Could you check a few things on this drawing? It's one solid part, dimensions in mm from its lowest x, y, z. A direction names the side the tool comes from. Give positions to 0.01 mm unless a question says otherwise; leave off trailing zeros. Write each loop counter-clockwise with the first axis right and the second up, starting at its lowest first coordinate (ties: lowest second). Pieces come first, ordered by that corner, then holes.
1. I'm going to push flat-ended pins straight in: pin 1 (5 mm diameter, centred on y = 19, z = 5, fed in from +X); pin 2 (1.5 mm diameter, centred on x = 4.5, z = 21, fed in from -Y); pin 3 (2 mm diameter, centred on x = 22.43, z = 25.97, fed in from -Y); pin 4 (0.8 mm diameter, centred on x = 5.5, y = 23.5, fed in from +Z) (1 decimal). Where does each tip first touch, or does it pass through?
2. On a 3-axis mill with a long thin cutter (end or side, diameter ignored), from which of +Z, -Z, +X, -X, +Y, -Y can I reach the whole of each face in a straight line? I mean the marked faces 1, 2 and 3. Say none if no direction works.
3. Thinking about a two-plate mould opening in X: for the marked faces 4, 5 and 6, which applies, pulls with the +X half, pulls with the -X half, needs draft (parallel to the pull), parting line crosses it, or undercut?
4. If I drill on probe 1 along Y at (x, z) = (1.5, 18.5); probe 2 along Y at (x, z) = (27.25, 16); probe 3 along Z at (x, y) = (15, 16.5), over which ranges is the centre line in solid material (lowest first)?
5. Suppose I cut it at C-C (z = 23). Please give me the cut outline in (x, y).
6. Suppose I cut it at B-B (x = 18). Please give me the cut outline in (y, z).
7. Suppose I cut it at A-A (z = 15). Please give me the cut outline in (x, y).
8. Suppose I cut it at D-D (y = 13). Please give me the cut outline in (x, z).
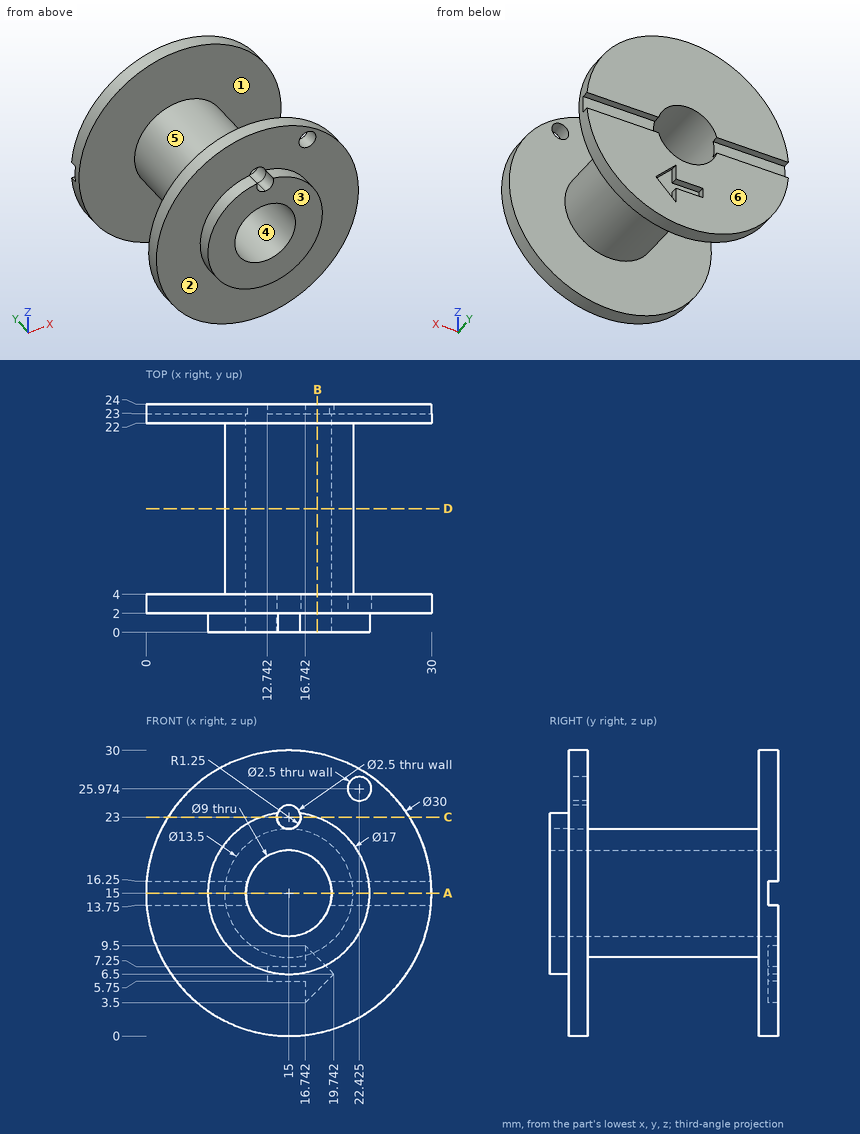
Checks:
1. pin 1: passes through
1. pin 2: stops at y = 2
1. pin 3: stops at y = 22
1. pin 4: stops at z = 26.9
2. face 1: none
2. face 2: -Y
2. face 3: +Z, -Z, +X, -X, -Y
3. face 4: undercut
3. face 5: parting line crosses it
3. face 6: needs draft
4. probe 1: y = 2 to 4, 22 to 24
4. probe 2: y = 2 to 4, 22 to 23
4. probe 3: z = 8.25 to 10.5, 19.5 to 21.75
5. outline: (2.31, 2) - (12.13, 2) - (12.13, 0) - (13.75, 0) - (13.75, 4) - (2.31, 4) - close; (2.31, 22) - (27.69, 22) - (27.69, 24) - (2.31, 24) - close; (16.25, 0) - (17.87, 0) - (17.87, 2) - (27.69, 2) - (27.69, 4) - (16.25, 4) - close
6. outline: (0, 7.05) - (2, 7.05) - (2, 0.3) - (4, 0.3) - (4, 8.95) - (22, 8.95) - (22, 0.3) - (24, 0.3) - (24, 4.76) - (23, 4.76) - (23, 8.24) - (24, 8.24) - (24, 11.65) - (0, 11.65) - close; (0, 18.35) - (24, 18.35) - (24, 29.7) - (22, 29.7) - (22, 21.05) - (4, 21.05) - (4, 29.7) - (2, 29.7) - (2, 22.95) - (0, 22.95) - close
7. outline: (0, 2) - (6.5, 2) - (6.5, 0) - (10.5, 0) - (10.5, 23) - (0, 23) - (0, 22) - (8.25, 22) - (8.25, 4) - (0, 4) - close; (19.5, 0) - (23.5, 0) - (23.5, 2) - (30, 2) - (30, 4) - (21.75, 4) - (21.75, 22) - (30, 22) - (30, 23) - (19.5, 23) - close
8. outline: circle Ø13.5 at (15, 15); hole circle Ø9 at (15, 15)
